Verification items for the finished model (mm, model axes). A direction names the side the tool comes from. Give positions to 0.01 mm unless a question says otherwise; leave off trailing zeros. Loops run counter-clockwise (first coordinate to the right, second up) from the corner with the lowest first, then second, coordinate; pieces in that order, holes last. Notation, with made-up numbers: (84, 36) - (124, 36) arc R27 cw to (124, 75) - close; hole circle Ø4 at (-18.75, -23.5). An arc over 180 degrees is marked (long way). One line per question, with ' | ' between items. Start each with the question number.
1. Section check B-B, the plane y = 0. Enter the section's corners in (x, z), then the cut area to 3 significant figures.
2. Depth check by flat-ended pin: pin 1 Ø1 at (x, y) = (-8, -1) entering from -Z; pin 2 Ø1 at (x, z) = (4, 1) entering from -Y; pin 3 Ø1 at (y, z) = (0, 0.5) entering from -X. Enter the tip coordinate at first touch or a pass-through.
3. Section check A-A, the plane z = 0. Enter the section's corners in (x, y), then the cut area to 3 significant figures.
4. Tool access check on faces 1 (the face through (-13.4, 1, 0)), 2 (the face through (-10.5, 0, 0)). Record the directions out of +Z, -Z, +X, -X, +Y, -Y that give a thin tool (end or side, any length) a straight path to the whole face; none if there is none.
5. Section check C-C, the plane x = -10. Enter the section's corners in (y, z).
6. Thickness scan on line 1 along X through (y, z) = (0.3, -0.95); line 2 along Y through (x, z) = (-11, 1.65); line 3 along Y through (x, z) = (4, 1.8). Record the ranges inside material, lowest first. Write a range as from..to.
Autodesk Inventor part; units mm, degrees
ref_plane "Work Plane3" through (-3.4, 0, 0) normal (0, 0, -1) x (1, 0, 0)
ref_plane "YZ Plane" through (0, 0, 0) normal (1, 0, 0) x (0, 1, 0)
ref_plane "XZ Plane" through (0, 0, 0) normal (0, 1, 0) x (-1, 0, 0)
sketch "Sketch1" plane through (0, 0, 0) normal (0, 0, 1) x (1, 0, 0)
  line L0 (0, 6.25) -> (0, -4.9479) construction
  line L1 (-13.4, 0) -> (-13.4, 3)
  line L2 (-13.4, 3) -> (6.6, 3)
  line L3 (6.6, 3) -> (6.6, 0)
  line L4 (-13.4, 0) -> (6.6, 0)
  line L5 (-17.4, 0) -> (10.6, 0)
  line L6 (0, 8.4896) -> (0, -7.1875)
  dimension "d0" = 6
  dimension "d1" = 6.6
  dimension "d2" = 20
revolve "Body" add sketch "Sketch1" angle 360 about axis through (-13.4, 0, 0) along (1, 0, 0)
sketch "Sketch2" plane through (-13.4, 0, 0) normal (-1, 0, 0) x (0, 0, 1)
  line L0 (0, -4.2) -> (0, 4.2)
  line L1 (-4.2, 0) -> (4.2, 0)
  line L2 (-3, 0.6) -> (3, 0.6)
  line L3 (3, 0.6) -> (3, -0.6)
  line L4 (3, -0.6) -> (-3, -0.6)
  line L5 (-3, -0.6) -> (-3, 0.6)
  line L6 (-3, 0) -> (3, 0) construction
  line L7 (0, 0.6) -> (0, -0.6) construction
  circle A0 centre (0, 0) radius 3
  dimension "d10" = 1.2
extrude "Slot" cut sketch "Sketch2" against normal blind 2.9 contours L4 A0 L1 L0 | L0 L1 A0 L4 | L4 L5 A0 | A0 L3 L4 | L1 A0 L2 L0 | L0 L2 A0 L1 | L5 L2 A0 | A0 L2 L3
chamfer "Chamfer1" distance 1 angle 45 3 edges at (-13.4, 2.3238, 1.8974) (-13.4, 2.3238, -1.8974) (-13.4, -3, 0) measured on face at (-6.7333, -3, 0)
thread "Thread"
chamfer "Chamfer2" distance 1 angle 45 1 edges at (6.6, -3, 0) measured on face at (-6.0667, -3, 0)
ref_plane "Work Plane3" through (-3.4, 0, 0) normal (0, 0, -1) x (1, 0, 0)
equation "\"d10\" = SBR"
equation "\"d11\" = STI"
equation "\"d4\" = PHH"
equation "\"d5\" = FAWI"
equation "\"d27\" = PHH"
equation "\"d6\" = GEL"
equation "\"d8\" = PHH"
equation "\"d9\" = FAWI"
equation "\"d0\" = NND"
equation "\"d1\" = GEL"
equation "\"d2\" = NLG"
equation "\"NND\" = 6"
equation "\"NLG\" = 20"
equation "\"PHH\" = 1"
equation "\"STI\" = 2.9"
equation "\"SBR\" = 1.2"
equation "\"GEL\" = 6.6"
equation "\"GD1\" = THREADDIA - 1.2269 * PTC"
equation "\"FAWI\" = 45deg"
equation "\"d14\" = -GEL"
equation "\"GUL\" = 0.61345 * PTC"
equation "\"THREADDIA\" = 6"
equation "\"TOA\" = 30deg"
equation "\"PTC\" = 1"
equation "\"GAL\" = 0.61345 * PTC"
properties part number "Pin GB 878-86 6 x 20" material "Steel, Mild"
Results list:
1) outline: (-10.5, -3) - (5.6, -3) - (6.6, -2) - (6.6, 2) - (5.6, 3) - (-10.5, 3) - close | area: 102 mm²
2) pin 1: z = -2.96 | pin 2: y = -2.96 | pin 3: x = -10.5
3) outline: (-13.4, -2) - (-12.4, -3) - (5.6, -3) - (6.6, -2) - (6.6, 2) - (5.6, 3) - (-12.4, 3) - (-13.4, 2) - (-13.4, 0.6) - (-10.5, 0.6) - (-10.5, -0.6) - (-13.4, -0.6) - close | area: 115 mm²
4) face 1: +Z, -Z, -X, +Y, -Y | face 2: +Z, -Z, -X
5) outline: circle Ø6 at (0, 0)
6) line 1: -10.5..6.6 | line 2: -2.51..-0.6, 0.6..2.51 | line 3: -2.4..2.4
